Autodesk Inventor part; units mm, degrees
ref_plane "YZ Plane" through (0, 0, 0) normal (1, 0, 0) x (0, 1, 0)
ref_plane "XZ Plane" through (0, 0, 0) normal (0, 1, 0) x (-1, 0, 0)
ref_plane "XY Plane" through (0, 0, 0) normal (0, 0, 1) x (1, 0, 0)
sketch "Sketch1" plane through (0, 0, 0) normal (0, 0, 1) x (1, 0, 0)
  line L0 (72.4944, 63.4773) -> (-72.5056, 63.4773)
  line L1 (72.4944, 63.4773) -> (-72.5232, -63.5025) construction
  line L2 (-72.5056, 63.4773) -> (72.5218, -63.4915) construction
  circle A0 centre (33.08, -58.41) radius 2.85
  line L3 (-72.5056, -38.1227) -> (-3.32, -68.51)
  line L4 (-72.5056, 63.4773) -> (-72.5056, -38.1227)
  line L5 (72.4944, 63.4773) -> (72.4944, -6.5227)
  line L6 (51.23, -68.51) -> (72.4944, -6.5227)
  line L7 (-3.32, -68.51) -> (51.23, -68.51)
  circle A1 centre (39.7605, -54.0088) radius 1.8
  circle A2 centre (28.6788, -51.7295) radius 1.8
  circle A3 centre (37.4812, -65.0905) radius 1.8
  circle A4 centre (26.3995, -62.8112) radius 1.8
  circle A5 centre (39.7605, -54.0088) radius 1.8
  circle A6 centre (37.4812, -65.0905) radius 1.8
  circle A7 centre (26.3995, -62.8112) radius 1.8
  circle A8 centre (28.6788, -51.7295) radius 1.8
  point P0 (0, 0)
  dimension "d6" = 145
  dimension "d9" = 70
extrude "Extrusion3" add sketch "Sketch1" along normal blind 3
properties part number "Bucket - door 2"
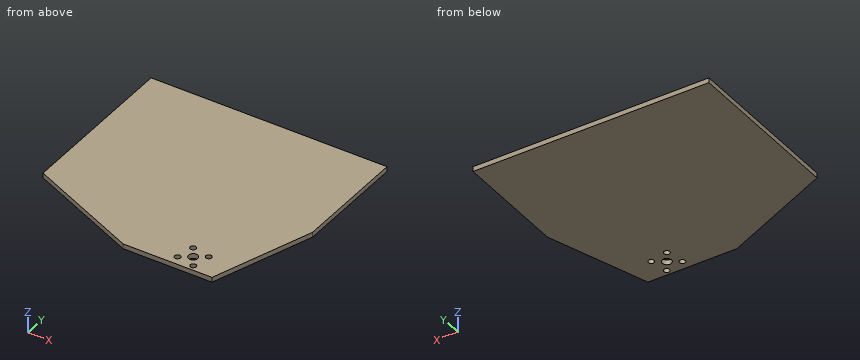
Geometry check sheet. Reference: the model listing, model coordinates, mm. Round coordinates to 2 decimals unless told otherwise and drop trailing zeros. Order: outer loops, then holes, each group sorted by start corner. A loop starts at its lowest first (then second) coordinate and runs counter-clockwise, first axis right, second up. Notation, with made-up numbers: M 45,25.5 L 68,25.5 A24 ccw 68,61.5 Z; hole C 69,30.5 d2. An arc over 180 degrees is marked long. Write item = value, one per line.
Q1. Section check C-C (z = 0.65). Enter the section's corners in (x, y).
Answer block:
outline = M -72.51,-38.12 L -3.32,-68.51 L 51.23,-68.51 L 72.49,-6.52 L 72.49,63.48 L -72.51,63.48 Z; hole C 26.4,-62.81 d3.6; hole C 28.68,-51.73 d3.6; hole C 33.08,-58.41 d5.7; hole C 37.48,-65.09 d3.6; hole C 39.76,-54.01 d3.6
Q2. Section check A-A (y = -58.41). Enter the section's corners in (x, z), plus the area to 3 significant figures.
Answer block:
outline = M -26.32,0 L 30.23,0 L 30.23,3 L -26.32,3 Z; M 35.93,0 L 54.69,0 L 54.69,3 L 35.93,3 Z
area = 226 mm^2
Q3. Scan lines: line 1 (Y direction, x = 33.08, z = 0.7); line 2 (X direction, y = -56.5, z = 2.6); line 3 (X direction, y = -55.5, z = 2.1). Record each from-to range of solid material in increasing order.
Answer block:
line_1 = -68.51 to -61.26, -55.56 to 63.48
line_2 = -30.66 to 30.96, 35.2 to 55.35
line_3 = -32.94 to 38.75, 40.77 to 55.69
Q4. Section check B-B (x = 33.08). Enter the section's corners in (y, z).
Answer block:
outline = M -68.51,0 L -61.26,0 L -61.26,3 L -68.51,3 Z; M -55.56,0 L 63.48,0 L 63.48,3 L -55.56,3 Z
Q5. Section check D-D (x = 57). Enter the section's corners in (y, z).
Answer block:
outline = M -51.69,0 L 63.48,0 L 63.48,3 L -51.69,3 Z
